```python
from build123d import *

# Parameters (mm, degrees)
F0_W     = 127
F0_H     = 127
F1_DEPTH = 25.4
F2_R     = 6.35
F3_T     = -5.08
F5_DEPTH = 2.54


with BuildPart() as f1:
    # F0 (on Top) → F1 (new body)
    with BuildSketch(Plane.XY):
        Rectangle(F0_W, F0_H)
    extrude(amount=F1_DEPTH)

    # F2
    f2_edges = [f1.edges().sort_by_distance(p)[0] for p in [
        (63.5, -63.5, 12.7),
        (63.5, 63.5, 12.7),
        (-63.5, 63.5, 12.7),
        (-63.5, -63.5, 12.7),
    ]]
    fillet(f2_edges, radius=F2_R)

    # F3
    f3_openings = [f1.faces().sort_by_distance(p)[0] for p in [
        (0, 0, 25.4),
    ]]
    offset(amount=F3_T, openings=f3_openings)

    # F4 (on face) → F5 (cut)
    with BuildSketch(Plane.XY.offset(25.4)):
        with BuildLine():
            Line((60.96, 60.96), (-57.785, 60.96))
            ThreePointArc((-57.785, 60.96), (-60.030064, 60.030064), (-60.96, 57.785))
            Line((-60.96, 57.785), (-60.96, -60.96))
            Line((-60.96, -60.96), (60.96, -60.96))
            Line((60.96, -60.96), (60.96, 60.96))
        make_face()
    extrude(amount=-F5_DEPTH, mode=Mode.SUBTRACT)


solid = f1.part
```
The listing builds one solid part. Answer for the finished solid, in the listing's coordinates (mm). A direction names the side the tool comes from. Coordinates: 2 decimals unless noted, no trailing zeros. Write each loop counter-clockwise with the first axis right and the second up, starting at its lowest first coordinate (ties: lowest second). Pieces come first, ordered by that corner, then holes.
Q1. Find the intervals of material crossed by line 1 along Y through (x, z) = (-56, 12.25); line 2 along Z through (x, y) = (-35.5, 27.5), in increasing order.
Returned:
line 1: y = -63.5 to -58.42, 58.42 to 63.5
line 2: z = 0 to 5.08
Q2. Given P1, Ø1, axis at x = 5.5, y = 25, coming from the -Z side; P2, Ø2, axis at x = -6, y = -46.5, coming from the +Z side, each flat-ended and moving along its own axis, determine where each tip first touches the part or whether it passes through.
Returned:
P1: stops at z = 0
P2: stops at z = 5.08
Q3. Section A-A, the plane x = -53 is taken. Write down the section's boundary in (y, z).
Returned:
outline: (-63.5, 0) - (63.5, 0) - (63.5, 25.4) - (60.96, 25.4) - (60.96, 22.86) - (58.42, 22.86) - (58.42, 5.08) - (-58.42, 5.08) - (-58.42, 22.86) - (-60.96, 22.86) - (-60.96, 25.4) - (-63.5, 25.4) - close
Q4. Section C-C, the plane z = 9.75 is taken. Write down the section's boundary in (x, y).
Returned:
outline: (-63.5, -57.15) arc R6.35 ccw to (-57.15, -63.5) - (57.15, -63.5) arc R6.35 ccw to (63.5, -57.15) - (63.5, 57.15) arc R6.35 ccw to (57.15, 63.5) - (-57.15, 63.5) arc R6.35 ccw to (-63.5, 57.15) - close; hole (-58.42, -57.15) arc R1.27 ccw to (-57.15, -58.42) - (57.15, -58.42) arc R1.27 ccw to (58.42, -57.15) - (58.42, 57.15) arc R1.27 ccw to (57.15, 58.42) - (-57.15, 58.42) arc R1.27 ccw to (-58.42, 57.15) - close
Q5. Which of the six approach directions +Z, -Z, +X, -X, +Y, -Y give full straight-line access (tool end or side, diameter ignored) to faces 1 (the cylindrical face through (61.69, 61.59, 12.88)), 2 (the flat face through (-1, 1, 5.08))?
Returned:
face 1: +Z, -Z, +X, +Y
face 2: +Z
